Could you check a few things on this model? Use its own coordinates, in mm. A direction names the side the tool comes from. Give positions to 0.01 mm unless a question says otherwise; leave off trailing zeros. Order: outer loops, then holes, each group sorted by start corner. A loop starts at its lowest first (then second) coordinate and runs counter-clockwise, first axis right, second up. Notation, with made-up numbers: (74.5, -25) -> (107.5, -25) arc R19 ccw to (107.5, -6) -> close; hole circle Ø8 at (-15, 14). An arc over 180 degrees is marked (long way). Answer as CSV lines item,"result". Start each with the question number.
(1) I need wall thicknesses on L1, parallel to X at y = -13, z = -43; L2, parallel to Y at x = 17, z = -35.5; L3, parallel to Z at x = 24, y = -1.5. Which ranges of each line are inside material? Lowest first, please.
(2) I want a section at A-A (z = -38.5). Please give me the cut outline in (x, y), plus the area to 3 significant figures.
(3) I want a section at C-C (x = 15.5). Please give me the cut outline in (y, z), plus the area to 4 significant figures.
(4) On a 3-axis mill with a long thin cutter (end or side, diameter ignored), from which of +Z, -Z, +X, -X, +Y, -Y can I reach the whole of each face in a straight line? I mean faces 4 (the face through (0, -8, -24)), 5 (the face through (15, 5, -4.139)), 6 (the face through (19, -12.795, -42)). Say none if no direction works.
(5) Will these pins go through, and if not, where does the flat tip stop? pin 1 Ø5 at (x, y) = (17.5, -19.5) entering from -Z; pin 2 Ø6 at (x, z) = (5.5, -11.5) entering from +Y.
(6) I want a section at D-D (x = 3.75). Please give me the cut outline in (y, z), plus the area to 4 significant figures.
(7) I want a section at B-B (y = 6). Please give me the cut outline in (x, z), plus the area to 3 significant figures.
(8) We'd pull the mould along Z, two halves only. Please class faces 1 (the face through (30, -8, -24)), 2 (the face through (15, -2.795, -16)), 3 (the face through (15, -8, 5.861)): released by +Z, released by -Z, zero draft, split by the parting line, or undercut.
Autodesk Inventor part; units mm, degrees
ref_plane "YZ Plane" through (0, 0, 0) normal (1, 0, 0) x (0, 1, 0)
ref_plane "XZ Plane" through (0, 0, 0) normal (0, 1, 0) x (-1, 0, 0)
ref_plane "XY Plane" through (0, 0, 0) normal (0, 0, 1) x (1, 0, 0)
sketch "Sketch1" plane through (0, 0, 0) normal (1, 0, 0) x (0, 1, 0)
  point P0 (0, 0)
sketch "Sketch2" plane through (0, 0, 0) normal (1, 0, 0) x (0, 1, 0)
  line L0 (12.2052, 5.8608) -> (-2.7948, 5.8608)
  line L1 (-2.7948, 5.8608) -> (-2.7948, -4.1392)
  line L2 (-2.7948, -4.1392) -> (12.2052, -4.1392)
  line L3 (12.2052, -4.1392) -> (12.2052, 5.8608)
  point P0 (0, 0)
  dimension "d0" = 15
  dimension "d1" = 10
extrude "Extrusion1" add sketch "Sketch2" along normal blind 30
sketch "Sketch3" plane through (30, 0, 0) normal (1, 0, 0) x (0, 0, -1)
  line L0 (-5.8608, -2.7948) -> (4.1392, -2.7948)
  line L1 (-5.8608, -2.7948) -> (54.1392, -2.7948)
  line L2 (54.1392, -2.7948) -> (54.1392, -27.7948)
  line L3 (54.1392, -27.7948) -> (-5.8608, -27.7948)
  line L4 (-5.8608, -27.7948) -> (-5.8608, -2.7948)
  point P0 (0, 0)
  dimension "d4" = 60
  dimension "d5" = 25
extrude "Extrusion2" add sketch "Sketch3" against normal blind 30
sketch "Sketch4" plane through (30, 0, 0) normal (1, 0, 0) x (0, 0, -1)
  line L0 (54.1392, -2.7948) -> (54.1392, -27.7948)
  line L1 (54.1392, -2.7948) -> (29.1392, -2.7948)
  line L2 (29.1392, -2.7948) -> (29.1392, 12.2052)
  line L3 (29.1392, 12.2052) -> (54.1392, 12.2052)
  line L4 (54.1392, 12.2052) -> (54.1392, -2.7948)
  point P0 (0, 0)
  dimension "d8" = 25
  dimension "d9" = 15
extrude "Extrusion3" add sketch "Sketch4" against normal blind 30
sketch "Sketch5" plane through (30, -27.7948, -54.1392) normal (0, 0, -1) x (-1, 0, 0)
  line L0 (0, 0) -> (30, 0)
  line L1 (0, 0) -> (0, 5)
  line L2 (0, 40) -> (0, 0)
  line L3 (0, 5) -> (3, 5)
  line L4 (3, 5) -> (18, 5)
  line L5 (18, 5) -> (18, 15)
  line L6 (18, 15) -> (3, 15)
  line L7 (3, 15) -> (3, 5)
  point P0 (30, 27.7948)
  dimension "d12" = 5
  dimension "d13" = 3
  dimension "d14" = 15
  dimension "d15" = 10
extrude "Extrusion4" cut sketch "Sketch5" against normal blind 25
Final values:
1,L1,"0 to 12, 27 to 30"
1,L2,"-27.79 to -22.79, -12.79 to 12.21"
1,L3,"-54.14 to -29.14, -4.14 to 5.86"
2,outline,"(0, -27.79) -> (30, -27.79) -> (30, 12.21) -> (0, 12.21) -> close; hole (12, -22.79) -> (27, -22.79) -> (27, -12.79) -> (12, -12.79) -> close"
2,area,"1,050 mm²"
3,outline,"(-27.79, -54.14) -> (-22.79, -54.14) -> (-22.79, -29.14) -> (-12.79, -29.14) -> (-12.79, -54.14) -> (12.21, -54.14) -> (12.21, -29.14) -> (-2.79, -29.14) -> (-2.79, -4.14) -> (12.21, -4.14) -> (12.21, 5.86) -> (-27.79, 5.86) -> close"
3,area,"1,775 mm²"
4,face 4,"+Z, -Z, -X, +Y, -Y"
4,face 5,"+X, -X, +Y"
4,face 6,"-Z"
5,pin 1,"z = -29.14"
5,pin 2,"y = -2.79"
6,outline,"(-27.79, -54.14) -> (12.21, -54.14) -> (12.21, -29.14) -> (-2.79, -29.14) -> (-2.79, -4.14) -> (12.21, -4.14) -> (12.21, 5.86) -> (-27.79, 5.86) -> close"
6,area,"2,025 mm²"
7,outline,"(0, -54.14) -> (30, -54.14) -> (30, -29.14) -> (0, -29.14) -> close; (0, -4.14) -> (30, -4.14) -> (30, 5.86) -> (0, 5.86) -> close"
7,area,"1,050 mm²"
8,face 1,"zero draft"
8,face 2,"undercut"
8,face 3,"released by +Z"
